CAD build for the part. Positions are in the model's coordinates, mm. Face numbers are marked on the shaded views. A direction names the side the tool comes from. Round coordinates to 2 decimals unless told otherwise and drop trailing zeros. Order: outer loops, then holes, each group sorted by start corner. A loop starts at its lowest first (then second) coordinate and runs counter-clockwise, first axis right, second up. Notation, with made-up numbers: M 50,-25 L 70,-25 A21 ccw 70,-19 Z; hole C 29.5,58 d3. An arc over 180 degrees is marked long. Answer as a JSON object with one key per item and string values.
```python
from build123d import *

# Parameters (mm, degrees)
BOSS_EXTRUDE1_DEPTH = 10
FILLET1_R           = 5
SKETCH3_W           = 60
SKETCH3_H           = 20
BOSS_EXTRUDE2_DEPTH = 60
FILLET2_R           = 20
SKETCH6_R           = 25
CUT_EXTRUDE1_DEPTH  = 271.0000001
SKETCH7_R           = 125
BOSS_EXTRUDE3_DEPTH = 60
SKETCH8_R           = 50
BOSS_EXTRUDE5_DEPTH = 59.9


with BuildPart() as part:
    # Sketch2 → Boss-Extrude1 (new body)
    with BuildSketch(Plane.XY):
        with BuildLine():
            Line((-140, 150), (140, 150))
            ThreePointArc((140, 150), (147.071067812, 147.071067812), (150, 140))
            Line((150, 140), (150, -140))
            ThreePointArc((150, -140), (147.071067812, -147.071067812), (140, -150))
            Line((140, -150), (-140, -150))
            ThreePointArc((-140, -150), (-147.071067812, -147.071067812), (-150, -140))
            Line((-150, -140), (-150, 140))
            ThreePointArc((-150, 140), (-147.071067812, 147.071067812), (-140, 150))
        make_face()
    extrude(amount=BOSS_EXTRUDE1_DEPTH)

    # Fillet1
    fillet1_edges = [part.edges().sort_by_distance(p)[0] for p in [
        (147.071067812, -147.071067812, 10),
        (150, 0, 10),
        (147.071067812, 147.071067812, 10),
        (0, 150, 10),
        (-147.071067812, 147.071067812, 10),
        (-150, 0, 10),
        (-147.071067812, -147.071067812, 10),
        (0, -150, 10),
    ]]
    fillet(fillet1_edges, radius=FILLET1_R)

    # Sketch3 → Boss-Extrude2 (add)
    with BuildSketch(Plane(origin=(0, 0, 0), x_dir=(-1, 0, 0), z_dir=(0, 0, -1))):
        with Locations((80, 110)):
            Rectangle(SKETCH3_W, SKETCH3_H)
        with Locations((-80, 110)):
            Rectangle(SKETCH3_W, SKETCH3_H)
        with Locations((80, -110)):
            Rectangle(SKETCH3_W, SKETCH3_H)
        with Locations((-80, -110)):
            Rectangle(SKETCH3_W, SKETCH3_H)
    extrude(amount=BOSS_EXTRUDE2_DEPTH)

    # Fillet2
    fillet2_edges = [part.edges().sort_by_distance(p)[0] for p in [
        (-110, 110, -60),
        (-50, 110, -60),
        (50, 110, -60),
        (110, 110, -60),
        (-50, -110, -60),
        (-110, -110, -60),
        (110, -110, -60),
        (50, -110, -60),
    ]]
    fillet(fillet2_edges, radius=FILLET2_R)

    # Sketch6 → Cut-Extrude1 (cut, through all)
    with BuildSketch(Plane.XZ.offset(120)):
        with Locations((-80, -30)):
            Circle(SKETCH6_R)
        with Locations((80, -30)):
            Circle(SKETCH6_R)
    extrude(amount=-CUT_EXTRUDE1_DEPTH, mode=Mode.SUBTRACT)

    # Sketch7 → Boss-Extrude3 (add)
    with BuildSketch(Plane.XY.offset(10)):
        Circle(SKETCH7_R)
    extrude(amount=BOSS_EXTRUDE3_DEPTH)

    # Sketch8 → Boss-Extrude5 (add)
    with BuildSketch(Plane.XY.offset(70)):
        Circle(SKETCH8_R)
    extrude(amount=BOSS_EXTRUDE5_DEPTH)


solid = part.part
```
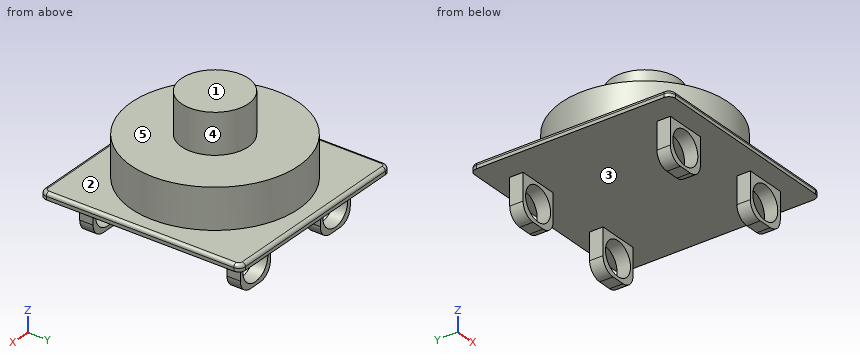
Item 1: Saw through at A-A on z = -30. State how many separate pieces and enclosed holes the cut face has, and give its area (3 significant figures).
Worked answers:
{"separate pieces": "8", "enclosed holes": "0", "area": "800 mm2"}
Item 2: Saw through at C-C on x = -80. List the corners of the cut face in (y, z), and give its area (3 significant figures).
Worked answers:
{"outline": "M -150,0 L -120,0 L -120,-5 L -100,-5 L -100,0 L 100,0 L 100,-5 L 120,-5 L 120,0 L 150,0 L 150,5 A5 ccw 145,10 L 96.05,10 L 96.05,70 L -96.05,70 L -96.05,10 L -145,10 A5 ccw -150,5 Z; M -120,-60 L -100,-60 L -100,-55 L -120,-55 Z; M 100,-60 L 120,-60 L 120,-55 L 100,-55 Z", "area": "14,900 mm2"}
Item 3: Wall check: line 1 along X through (y, z) = (-106, -28.5); line 2 along Z through (x, y) = (80, -108.25); line 3 along Z through (x, y) = (-79, -21). Give the ranges that are in metal, low to high. Write a range as [from, to].
Worked answers:
{"line 1": "x = [-110, -104.95], [-55.05, -50], [50, 55.05], [104.95, 110]", "line 2": "z = [-60, -55], [-5, 10]", "line 3": "z = [0, 70]"}
Item 4: 3-axis set-ups, long thin cutter, end or side, ignore diameter. For the marked faces 1 and 2: which of +Z, -Z, +X, -X, +Y, -Y reach the whole face in a straight line?
Worked answers:
{"face 1": "+Z, +X, -X, +Y, -Y", "face 2": "+Z"}
Item 5: Saw through at B-B on y = 0. List the corners of the cut face in (x, z).
Worked answers:
{"outline": "M -150,0 L 150,0 L 150,5 A5 ccw 145,10 L 125,10 L 125,70 L 50,70 L 50,129.9 L -50,129.9 L -50,70 L -125,70 L -125,10 L -145,10 A5 ccw -150,5 Z"}
Item 6: Drop flat-ended pins along their axis: pin 1 Ø16 at (y, z) = (-113, -16) entering from +X; pin 2 Ø8 at (x, y) = (-46.5, 62) entering from +Z; pin 3 Ø16 at (y, z) = (109.5, -25) entering from -X; pin 4 Ø18 at (x, z) = (-68.5, -19.5) entering from -Y. Give the stop position or say it passes through.
Worked answers:
{"pin 1": "stops at x = 110", "pin 2": "stops at z = 70", "pin 3": "stops at x = -110", "pin 4": "passes through"}
Item 7: Two-plate mould, pull along Y, no slides. Class the marked faces 3, 4 and 5: released by +Y, released by -Y, zero draft, split by the parting line, or undercut.
Worked answers:
{"face 3": "undercut", "face 4": "split by the parting line", "face 5": "zero draft"}
